Check sheet for the modelled part. Datum: model origin and axes. Units: mm. Give positions to 0.01 mm unless a question says otherwise; leave off trailing zeros. Order: outer loops, then holes, each group sorted by start corner. A loop starts at its lowest first (then second) coordinate and runs counter-clockwise, first axis right, second up.
```python
from build123d import *

# Parameters (mm, degrees)
Y_KSEKLIK_EKSTR_ZYON3_DEPTH = 200


with BuildPart() as part:
    # Model → Yükseklik-Ekstrüzyon3 (new body)
    with BuildSketch(Plane.XY):
        with BuildLine():
            Line((-4.75, 21), (-4.75, 24.442739208))
            ThreePointArc((-4.75, 24.442739208), (-24.9, 0), (-4.75, -24.442739208))
            Line((-4.75, -24.442739208), (-4.75, -21))
            ThreePointArc((-4.75, -21), (-4.530330086, -20.469669914), (-4, -20.25))
            Line((-4, -20.25), (0, -20.25))
            Line((0, -20.25), (4, -20.25))
            ThreePointArc((4, -20.25), (4.530330086, -20.469669914), (4.75, -21))
            Line((4.75, -21), (4.75, -24.442739208))
            ThreePointArc((4.75, -24.442739208), (24.9, 0), (4.75, 24.442739208))
            Line((4.75, 24.442739208), (4.75, 21))
            ThreePointArc((4.75, 21), (4.530330086, 20.469669914), (4, 20.25))
            Line((4, 20.25), (0, 20.25))
            Line((0, 20.25), (-4, 20.25))
            ThreePointArc((-4, 20.25), (-4.530330086, 20.469669914), (-4.75, 21))
        make_face()
    extrude(amount=Y_KSEKLIK_EKSTR_ZYON3_DEPTH)


solid = part.part
```
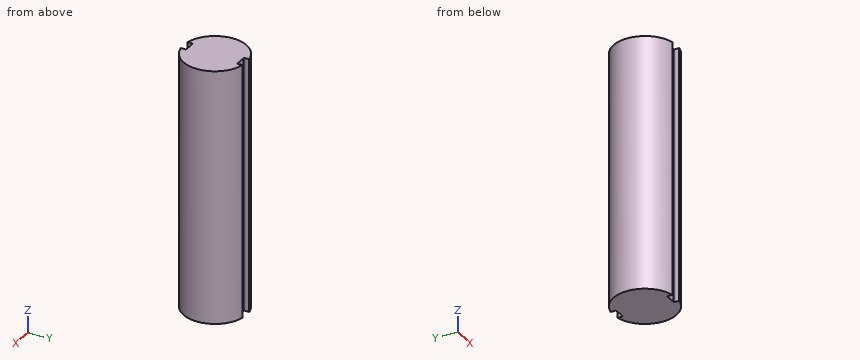
(1) Cross-section at A-A on z = 172.5. Enter the section's corners in (x, y).
Response values:
outline: (-4.75, -24.44) - (-4.75, -21) arc R0.75 cw to (-4, -20.25) - (4, -20.25) arc R0.75 cw to (4.75, -21) - (4.75, -24.44) arc R24.9 ccw to (4.75, 24.44) - (4.75, 21) arc R0.75 cw to (4, 20.25) - (-4, 20.25) arc R0.75 cw to (-4.75, 21) - (-4.75, 24.44) arc R24.9 ccw to start
(2) Material ranges on L1, parallel to X at y = 20.5, z = 131; L2, parallel to Y at x = 4, z = 141, recorded low to high.
Response values:
L1: x = -14.13 to -4.56, 4.56 to 14.13
L2: y = -20.25 to 20.25
(3) Gauge pin test, flat ends, axial feed: pin 1 Ø4 at (y, z) = (22, 72) entering from +X; pin 2 Ø8 at (x, z) = (18.5, 171) entering from -Y; pin 3 Ø3 at (y, z) = (23, 124) entering from -X. Record the tip position at first contact, or that the pin passes through.
Response values:
pin 1: stops at x = 14.83
pin 2: stops at y = -20.24
pin 3: stops at x = -12.56
(4) Cross-section at C-C on y = 10. Enter the section's corners in (x, z), then the cut area to 3 significant figures.
Response values:
outline: (-22.8, 0) - (22.8, 0) - (22.8, 200) - (-22.8, 200) - close
area: 9,120 mm2
(5) Cross-section at B-B on x = 0.5. Enter the section's corners in (y, z), then the cut area to 3 significant figures.
Response values:
outline: (-20.25, 0) - (20.25, 0) - (20.25, 200) - (-20.25, 200) - close
area: 8,100 mm2
